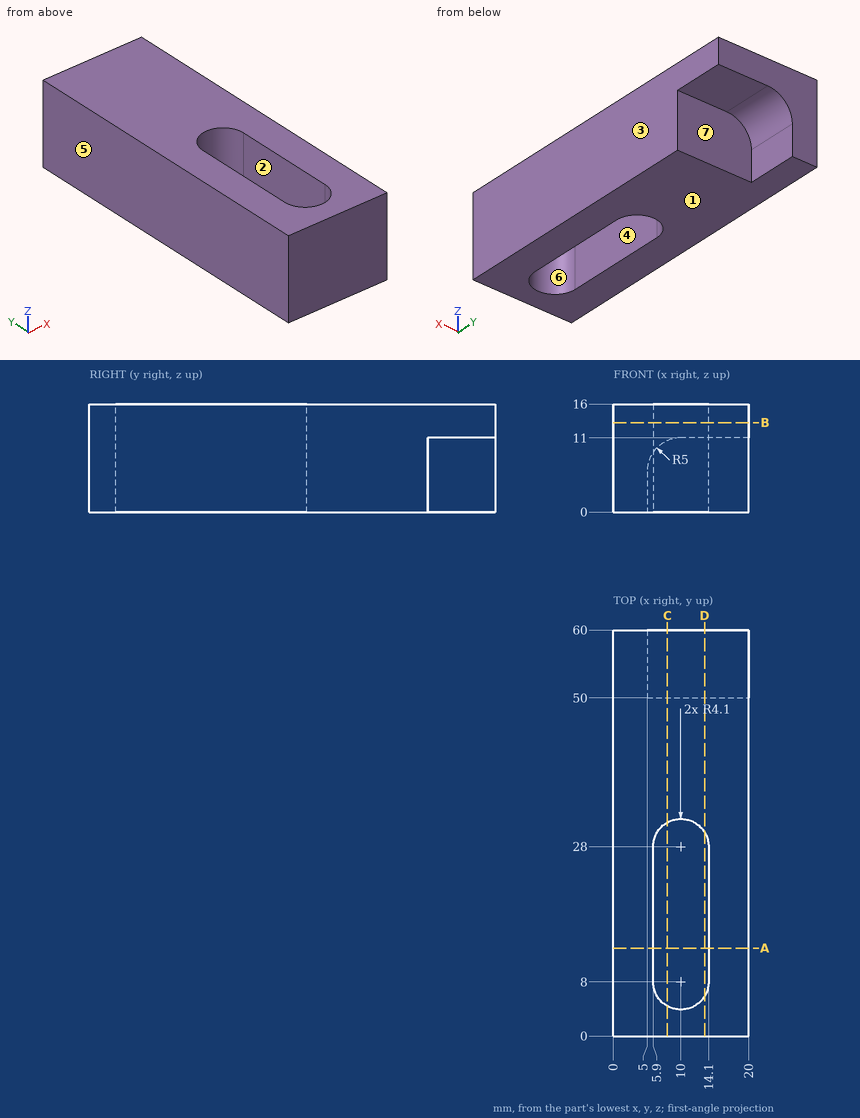
The drawing under review shows one solid part. Ordinate dimensions are in mm from its lowest x, y, z. A direction names the side the tool comes from. Give positions to 0.01 mm unless a question says otherwise; leave off trailing zeros. Write each loop counter-clockwise with the first axis right and the second up, starting at its lowest first coordinate (ties: lowest second). Pieces come first, ordered by that corner, then holes. Notation, with made-up numbers: (-39.5, -27) -> (-14.5, -27) arc R21 ccw to (-14.5, 10) -> close; hole circle Ø11 at (15.25, -32). An arc over 180 degrees is marked (long way). Put each result on its own line as item: value.
(1) We need section A-A, the plane y = 13. Give the boundary of the cut face in (x, z).
Results are:
outline: (0, 0) -> (5.9, 0) -> (5.9, 16) -> (0, 16) -> close; (14.1, 0) -> (20, 0) -> (20, 16) -> (14.1, 16) -> close
(2) To check wall thickness, follow probe 1 along X at (y, z) = (23, 11); probe 2 along Y at (x, z) = (16.25, 5.75); probe 3 along Y at (x, z) = (11, 9.75). State the ranges of each line that lie inside material, in increasing order. Write a range as from..to.
Results are:
probe 1: 0..5.9, 14.1..20
probe 2: 0..50
probe 3: 0..4.02, 31.98..50
(3) The part is to be moulded in two halves that separate along X. For the marked faces 1, 2, 3 and 4, say which applies: pulls with the +X half, pulls with the -X half, needs draft (parallel to the pull), parting line crosses it, or undercut.
Results are:
face 1: needs draft
face 2: undercut
face 3: pulls with the +X half
face 4: undercut
(4) We need section B-B, the plane z = 13.25. Give the boundary of the cut face in (x, y), and give its area (3 significant figures).
Results are:
outline: (0, 0) -> (20, 0) -> (20, 60) -> (0, 60) -> close; hole (5.9, 8) arc R4.1 ccw to (14.1, 8) -> (14.1, 28) arc R4.1 ccw to (5.9, 28) -> close
area: 983 mm²
(5) Tool access review of the marked faces 5, 6 and 7: name each direction out of +Z, -Z, +X, -X, +Y, -Y from which nothing blocks a thin tool from reaching the whole face with its end or side.
Results are:
face 5: +Z, -Z, -X, +Y, -Y
face 6: +Z, -Z
face 7: -Z, +X, +Y
(6) We need section D-D, the plane x = 13.5. Give the boundary of the cut face in (y, z), and give its area (3 significant figures).
Results are:
outline: (0, 0) -> (5.86, 0) -> (5.86, 16) -> (0, 16) -> close; (30.14, 0) -> (50, 0) -> (50, 11) -> (60, 11) -> (60, 16) -> (30.14, 16) -> close
area: 462 mm²
(7) For pin 1 Ø6.5 at (y, z) = (55, 2.5) entering from +X; pin 2 Ø5 at (x, y) = (12.5, 53.5) entering from -Z; pin 3 Ø5.5 at (x, z) = (13.5, 6) entering from +Y; pin 4 Ø1 at (x, y) = (8, 13) entering from -Z, all flat-tipped, find the tip position at first contact; note any pin that passes through.
Results are:
pin 1: x = 5
pin 2: z = 11
pin 3: y = 50
pin 4: through
(8) We need section C-C, the plane x = 8. Give the boundary of the cut face in (y, z).
Results are:
outline: (0, 0) -> (4.42, 0) -> (4.42, 16) -> (0, 16) -> close; (31.58, 0) -> (50, 0) -> (50, 10.58) -> (60, 10.58) -> (60, 16) -> (31.58, 16) -> close
